```python
from build123d import *

# Parameters (mm, degrees)
BASE_FLANGE1_DEPTH     = 2
TAB1_START             = -2
TAB1_OUTLINE_W         = 950
TAB1_OUTLINE_H         = 35
TAB1_DEPTH             = 2
SKETCHED_START         = -950
SKETCHED_BEND1_DEPTH   = 950
SKETCHED_BEND1_2_DEPTH = 950
FILLET1_R              = 0.78
FILLET2_R              = 0.74
SKETCH10_R             = 4
CUT_EXTRUDE1_DEPTH     = 10


# Read off the part's stored shape, not the designer's step: Tab1, Sketched Bend1
# Sheet-metal steps are written as plain solids
with BuildPart() as part:
    # Sketch1 → Base-Flange1 (new body)
    with BuildSketch(Plane(origin=(0, 0, 0), x_dir=(0, 0, -1), z_dir=(1, 0, 0))):
        Polygon((0, 0), (0, -300), (650, -550), (950, -550), (950, 0), align=None)
    extrude(amount=-BASE_FLANGE1_DEPTH)

    # Tab1 outline → Tab1 (add)
    with BuildSketch(Plane(origin=(0, 0, 0), x_dir=(0, 0, -1), z_dir=(1, 0, 0)).offset(TAB1_START)):
        with Locations((475, 17.5)):
            Rectangle(TAB1_OUTLINE_W, TAB1_OUTLINE_H)
    extrude(amount=TAB1_DEPTH)

    # Sketched Bend1 outline → Sketched Bend1 (cut)
    with BuildSketch(Plane.XY.offset(SKETCHED_START)):
        with BuildLine():
            Line((-2, 35), (-2, 2.635602398))
            ThreePointArc((-2, 2.635602398), (-0.556604688, 1.654267209), (0, 0))
            Line((0, 0), (0, 35))
            Line((0, 35), (-2, 35))
        make_face()
    extrude(amount=SKETCHED_BEND1_DEPTH, mode=Mode.SUBTRACT)

    # Sketched Bend1 2 outline → Sketched Bend1 2 (add)
    with BuildSketch(Plane.XY.offset(SKETCHED_START)):
        with BuildLine():
            Line((-35.008755099, 0.7366), (-2.7366, 0.7366))
            ThreePointArc((-2.7366, 0.7366), (-2.215745145, 0.520854855), (-2, 0))
            Line((-2, 0), (-2, 2.635602398))
            ThreePointArc((-2, 2.635602398), (-2.364854094, 2.711233029), (-2.7366, 2.7366))
            Line((-2.7366, 2.7366), (-35.008755099, 2.7366))
            Line((-35.008755099, 2.7366), (-35.008755099, 0.7366))
        make_face()
    extrude(amount=SKETCHED_BEND1_2_DEPTH)

    # Fillet1
    fillet1_edges = [part.edges().sort_by_distance(p)[0] for p in [
        (-1, -300, 0),
    ]]
    fillet(fillet1_edges, radius=FILLET1_R)

    # Fillet2
    fillet2_edges = [part.edges().sort_by_distance(p)[0] for p in [
        (-1, -550, -650),
    ]]
    fillet(fillet2_edges, radius=FILLET2_R)

    # Sketch10 → Cut-Extrude1 (cut)
    with BuildSketch(Plane.XZ.offset(-0.7366)):
        with Locations((-18.872677549, -25)):
            Circle(SKETCH10_R)
        with Locations((-18.872677549, -125)):
            Circle(SKETCH10_R)
        with Locations((-18.872677549, -225)):
            Circle(SKETCH10_R)
        with Locations((-18.872677549, -325)):
            Circle(SKETCH10_R)
        with Locations((-18.872677549, -425)):
            Circle(SKETCH10_R)
        with Locations((-18.872677549, -525)):
            Circle(SKETCH10_R)
        with Locations((-18.872677549, -625)):
            Circle(SKETCH10_R)
        with Locations((-18.872677549, -725)):
            Circle(SKETCH10_R)
        with Locations((-18.872677549, -825)):
            Circle(SKETCH10_R)
        with Locations((-18.872677549, -925)):
            Circle(SKETCH10_R)
    extrude(amount=-CUT_EXTRUDE1_DEPTH, mode=Mode.SUBTRACT)


solid = part.part
```
The listing builds one solid part. Answer for the finished solid, in the listing's coordinates (mm). A direction names the side the tool comes from. Give positions to 0.01 mm unless a question says otherwise; leave off trailing zeros. Order: outer loops, then holes, each group sorted by start corner. A loop starts at its lowest first (then second) coordinate and runs counter-clockwise, first axis right, second up.
Item 1: Given pin 1 Ø10 at (y, z) = (-432, -562) entering from -X; pin 2 Ø13 at (x, z) = (-18.87, -125) entering from -Y, each flat-ended and moving along its own axis, determine where each tip first touches the part or whether it passes through.
From the geometry:
pin 1: stops at x = -2
pin 2: stops at y = 0.74
Item 2: The part is cut by section B-B, the plane x = -8.5. Give the vertices of the cut face in (y, z).
From the geometry:
outline: (0.74, -950) - (2.74, -950) - (2.74, 0) - (0.74, 0) - close
Item 3: The part is cut by section C-C, the plane y = -45. Give the vertices of the cut face in (x, z), and give its area (3 significant figures).
From the geometry:
outline: (-2, -950) - (0, -950) - (0, 0) - (-2, 0) - close
area: 1,900 mm2
Item 4: The part is cut by section A-A, the plane z = -886.5. Give the vertices of the cut face in (x, y), and give its area (3 significant figures).
From the geometry:
outline: (-35.01, 0.74) - (-2.74, 0.74) arc R0.74 cw to (-2, 0) - (-2, -550) - (0, -550) - (0, 0) arc R2.74 ccw to (-2.74, 2.74) - (-35.01, 2.74) - close
area: 1,170 mm2
Item 5: Find the intervals of material crossed by probe 1 along X at (y, z) = (1.5, -625); probe 2 along X at (y, z) = (1, -425); probe 3 along Y at (x, z) = (-9, -802), in increasing order.
From the geometry:
probe 1: x = -35.01 to -22.87, -14.87 to -0.45
probe 2: x = -35.01 to -22.87, -14.87 to -0.19
probe 3: y = 0.74 to 2.74
Item 6: The part is cut by section D-D, the plane z = -278. Give the vertices of the cut face in (x, y), and give its area (3 significant figures).
From the geometry:
outline: (-35.01, 0.74) - (-2.74, 0.74) arc R0.74 cw to (-2, 0) - (-2, -406.92) - (0, -406.92) - (0, 0) arc R2.74 ccw to (-2.74, 2.74) - (-35.01, 2.74) - close
area: 884 mm2
Item 7: Which of the six approach directions +Z, -Z, +X, -X, +Y, -Y give full straight-line access (tool end or side, diameter ignored) to faces 1 (the face through (-0.986, -423.323, -320.64)), 2 (the face through (-2, -210, -468))?
From the geometry:
face 1: +Z, +X, -X, -Y
face 2: +Z, -Z, -X, -Y
